Read the model definition and answer for the solid it produces. Units are mm, in the model's axes. A direction names the side the tool comes from. Round coordinates to 2 decimals unless told otherwise and drop trailing zeros. Order: outer loops, then holes, each group sorted by start corner. A loop starts at its lowest first (then second) coordinate and runs counter-clockwise, first axis right, second up. Notation, with made-up numbers: (17.5, -40) -> (26.5, -40) arc R6 cw to (26.5, -32) -> close; hole circle Ø6 at (41.5, -4). An arc over 180 degrees is marked (long way). Answer as a JSON object with one key per item and string values. Group by question number.
Item 1: Section A-A, the plane z = 20 is taken. Count the separate pieces of the cut face and the enclosed holes in it, plus the area to 3 significant figures.
Item 2: For faces 1 (the cylindrical face through (0, 4, 20)), 2 (the flat face through (61, 4, 27)), determine the directions among +Z, -Z, +X, -X, +Y, -Y from which every point of the face is accessible in a straight line to the end or side of a thin tool.
Item 3: Given P1, Ø4, axis at x = 63.5, z = 4, coming from the +Y side; P2, Ø2, axis at y = 8, z = 20, coming from the -X side; P3, Ø5, axis at y = 4.5, z = 10.5, coming from the -X side (3 decimals), each flat-ended and moving along its own axis, determine where each tip first touches the part or whether it passes through.
Item 4: Section B-B, the plane y = 21.5 is taken. Write down the section's boundary in (x, z).
Item 5: Consider probe 1 along Z at (x, y) = (23, 3); probe 2 along X at (y, z) = (19, 24.5); probe 3 along Z at (x, y) = (12, 1). Determine where each line is inside the solid, lowest interval first. Write a range as from..to.
Item 6: Section C-C, the plane y = 13.75 is taken. Write down the section's boundary in (x, z), plus the area to 3 significant figures.
from build123d import *

# Parameters (mm, degrees)
SALIENTE_EXTRUIR1_DEPTH = 8
CROQUIS2_R              = 20
SALIENTE_EXTRUIR2_DEPTH = 15
SALIENTE_EXTRUIR2_TAPER = 13
CROQUIS4_R              = 8
CORTAR_EXTRUIR3_DEPTH   = 23
CORTAR_EXTRUIR3_TAPER   = -10


with BuildPart() as part:
    # Croquis1 → Saliente-Extruir1 (new body)
    with BuildSketch(Plane(origin=(0, 0, 0), x_dir=(1, 0, 0), z_dir=(0, 1, 0))):
        with BuildLine():
            Line((20, 0), (80, 0))
            Line((80, 0), (80, -40))
            Line((80, -40), (20, -40))
            ThreePointArc((20, -40), (0, -20), (20, 0))
        make_face()
        with BuildLine():
            Line((68, -13), (54, -13))
            ThreePointArc((54, -13), (47, -20), (54, -27))
            Line((54, -27), (68, -27))
            ThreePointArc((68, -27), (75, -20), (68, -13))
        make_face(mode=Mode.SUBTRACT)
    extrude(amount=SALIENTE_EXTRUIR1_DEPTH)

    # Croquis2 → Saliente-Extruir2 (add)
    with BuildSketch(Plane(origin=(0, 8, 0), x_dir=(1, 0, 0), z_dir=(0, 1, 0))):
        with Locations((20, -20)):
            Circle(CROQUIS2_R)
    extrude(amount=SALIENTE_EXTRUIR2_DEPTH, taper=SALIENTE_EXTRUIR2_TAPER)

    # Croquis4 → Cortar-Extruir3 (cut)
    with BuildSketch(Plane(origin=(0, 23, 0), x_dir=(1, 0, 0), z_dir=(0, 1, 0))):
        with Locations((20, -20)):
            Circle(CROQUIS4_R)
    extrude(amount=-CORTAR_EXTRUIR3_DEPTH, taper=CORTAR_EXTRUIR3_TAPER, mode=Mode.SUBTRACT)


solid = part.part
Values found:
{
 "1": {"separate pieces": "3", "enclosed holes": "0", "area": "503 mm2"},
 "2": {"face 1": "-X, +Y, -Y", "face 2": "+Y, -Y"},
 "3": {"P1": "y = 8", "P2": "x = 0", "P3": "x = 1.265"},
 "4": {"outline": "circle Ø33.77 at (20, 20); hole circle Ø16.53 at (20, 20)"},
 "5": {"probe 1": "0..8.87, 31.13..40", "probe 2": "3.13..12.55, 27.45..36.87", "probe 3": "1.67..11.22, 28.78..38.33"},
 "6": {"outline": "circle Ø37.35 at (20, 20); hole circle Ø19.26 at (20, 20)", "area": "804 mm2"}
}
